Part model, mm, in its own coordinate system. Coordinates: 2 decimals unless noted, no trailing zeros. Write each loop counter-clockwise with the first axis right and the second up, starting at its lowest first coordinate (ties: lowest second). Pieces come first, ordered by that corner, then holes. Notation, with made-up numbers: M 30.5,5 L 69.5,5 A18 ccw 69.5,16 Z; hole C -35,55 d1. An arc over 180 degrees is marked long. Use a Markdown table: item, result. Add a question column.
Q1. Slice it at D-D on x = -24. Write the cut outline in (y, z), then the cut area to 3 significant figures.
Q2. Slice it at B-B on y = 0.5. Write the cut outline in (x, z), then the cut area to 3 significant figures.
Q3. Pin check, flat tips, straight feed: pin 1 Ø1.5 at (x, z) = (-14, -3.5) entering from -Y; pin 2 Ø1 at (y, z) = (0.5, -2.5) entering from -X. Stop position of each tip, or through.
Q4. Slice it at C-C on z = -2.25. Write the cut outline in (x, y).
Q5. Slice it at A-A on x = 0. Write the cut outline in (y, z).
Q6. Wall check: L1, parallel to X at y = 1.35, z = 11.25; L2, parallel to Z at x = 14.5, y = 1.3; L3, parallel to X at y = 1, z = 0. Give the ranges that are in metal, low to high. Write a range as from..to.
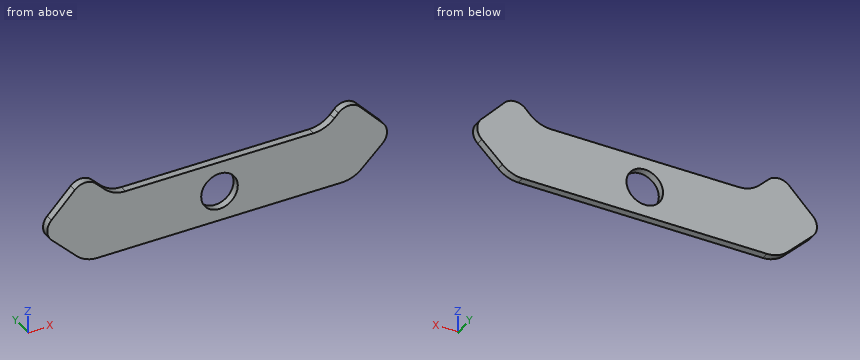
from build123d import *

# Parameters (mm, degrees)
SKETCH2_R           = 4.868124445
BOSS_EXTRUDE1_DEPTH = 2


with BuildPart() as part:
    # Sketch2 → Boss-Extrude1 (new body)
    with BuildSketch(Plane(origin=(0, 0, 0), x_dir=(1, 0, 0), z_dir=(0, 1, 0))):
        with BuildLine():
            ThreePointArc((37.278070291, -11.408685578), (34.482702596, -12.629587927), (31.664894392, -11.461409849))
            Line((31.664894392, -11.461409849), (30.562457969, -10.336699734))
            ThreePointArc((30.562457969, -10.336699734), (28.016666385, -8.607896753), (25, -8))
            Line((25, -8), (-25, -8))
            ThreePointArc((-25, -8), (-27.944700918, -8.578087681), (-30.452299379, -10.226541143))
            Line((-30.452299379, -10.226541143), (-32.975396929, -12.699671418))
            ThreePointArc((-32.975396929, -12.699671418), (-35.740493562, -13.812747241), (-38.482775603, -12.644592123))
            Line((-38.482775603, -12.644592123), (-44.703876064, -6.297800167))
            ThreePointArc((-44.703876064, -6.297800167), (-45.816951887, -3.532703535), (-44.648796769, -0.790421493))
            Line((-44.648796769, -0.790421493), (-37.952299379, 5.773458857))
            ThreePointArc((-37.952299379, 5.773458857), (-35.444700918, 7.421912319), (-32.5, 8))
            Line((-32.5, 8), (32.5, 8))
            ThreePointArc((32.5, 8), (35.376842294, 7.449252444), (37.846850837, 5.874894716))
            Line((37.846850837, 5.874894716), (43.341622103, 0.687699611))
            ThreePointArc((43.341622103, 0.687699611), (44.561082794, -2.032155678), (43.500143599, -4.817672722))
            Line((43.500143599, -4.817672722), (37.278070291, -11.408685578))
        make_face()
        with Locations(Location((0, 0, 0), (0, 0, 270))):
            Circle(SKETCH2_R, mode=Mode.SUBTRACT)
    extrude(amount=BOSS_EXTRUDE1_DEPTH)


solid = part.part
Recorded:
| question | item | result |
|---|---|---|
| 1 | outline | M 0,-8 L 2,-8 L 2,8 L 0,8 Z |
| 1 | area | 32.0 mm² |
| 2 | outline | M -44.7,6.3 A3.89 ccw -44.65,0.79 L -37.95,-5.77 A7.79 ccw -32.5,-8 L 32.5,-8 A7.79 ccw 37.85,-5.87 L 43.34,-0.69 A3.89 ccw 43.5,4.82 L 37.28,11.41 A3.89 ccw 31.66,11.46 L 30.56,10.34 A7.79 cw 25,8 L -25,8 A7.79 cw -30.45,10.23 L -32.98,12.7 A3.89 ccw -38.48,12.64 Z; hole C 0,0 d9.74 |
| 2 | area | 1,360 mm² |
| 3 | pin 1 | y = 0 |
| 3 | pin 2 | x = -41.8 |
| 4 | outline | M -41.55,0 L -4.32,0 L -4.32,2 L -41.55,2 Z; M 4.32,0 L 41.69,0 L 41.69,2 L 4.32,2 Z |
| 5 | outline | M 0,-8 L 2,-8 L 2,-4.87 L 0,-4.87 Z; M 0,4.87 L 2,4.87 L 2,8 L 0,8 Z |
| 6 | L1 | -39.85..-31.5, 31.46..37.43 |
| 6 | L2 | -8..8 |
| 6 | L3 | -43.84..-4.87, 4.87..43.92 |
